from build123d import *

# Parameters (mm, degrees)
BOSS_EXTRUDE1_DEPTH = 4.8
SKETCH2_R           = 8.5
BOSS_EXTRUDE2_DEPTH = 8.5
CUT_EXTRUDE1_DEPTH  = 18.927353402


with BuildPart() as part:
    # Sketch1 → Boss-Extrude1 (new body)
    with BuildSketch(Plane(origin=(0, 0, 0), x_dir=(1, 0, 0), z_dir=(0, 1, 0))):
        Polygon((-6, 3.464101615), (0, 6.92820323), (6, 3.464101615), (6, -3.464101615), (0, -6.92820323), (-6, -3.464101615), align=None)
    extrude(amount=BOSS_EXTRUDE1_DEPTH)

    # Sketch2 → Boss-Extrude2 (add)
    with BuildSketch(Plane(origin=(0, 4.8, 0), x_dir=(1, 0, 0), z_dir=(0, 1, 0))):
        with Locations(Location((0, 0, 0), (0, 0, 270))):
            Circle(SKETCH2_R)
    extrude(amount=BOSS_EXTRUDE2_DEPTH)

    # Sketch3 → Cut-Extrude1 (cut, through all)
    with BuildSketch(Plane(origin=(0, 13.3, 0), x_dir=(1, 0, 0), z_dir=(0, 1, 0))):
        with BuildLine():
            Line((-1.802775638, 3), (1.802775638, 3))
            ThreePointArc((1.802775638, 3), (0, -3.5), (-1.802775638, 3))
        make_face()
    extrude(amount=-CUT_EXTRUDE1_DEPTH, mode=Mode.SUBTRACT)


solid = part.part
Verification items for the finished model (mm, model axes). A direction names the side the tool comes from. Round coordinates to 2 decimals unless told otherwise and drop trailing zeros. Order: outer loops, then holes, each group sorted by start corner. A loop starts at its lowest first (then second) coordinate and runs counter-clockwise, first axis right, second up.
1. Section check B-B on y = 4.5. Record the cut outline in (x, z), then the cut area to 3 significant figures.
Final values:
outline: (-6, -3.46) - (0, -6.93) - (6, -3.46) - (6, 3.46) - (0, 6.93) - (-6, 3.46) - close; hole (-1.8, -3) - (1.8, -3) arc R3.5 ccw (long way) to start
area: 87.4 mm2
2. Thickness scan on L1, parallel to X at y = 8.25, z = 0; L2, parallel to Y at x = 0.25, z = 7; L3, parallel to Z at x = 0.75, y = 12.5. Record the ranges inside material, lowest first.
Final values:
L1: x = -8.5 to -3.5, 3.5 to 8.5
L2: y = 4.8 to 13.3
L3: z = -8.47 to -3, 3.42 to 8.47
3. Section check C-C on x = 2.25. Record the cut outline in (y, z).
Final values:
outline: (0, -5.63) - (4.8, -5.63) - (4.8, -8.2) - (13.3, -8.2) - (13.3, -2.68) - (0, -2.68) - close; (0, 2.68) - (13.3, 2.68) - (13.3, 8.2) - (4.8, 8.2) - (4.8, 5.63) - (0, 5.63) - close
4. Section check A-A on z = 0. Record the cut outline in (x, y), then the cut area to 3 significant figures.
Final values:
outline: (-8.5, 4.8) - (-6, 4.8) - (-6, 0) - (-3.5, 0) - (-3.5, 13.3) - (-8.5, 13.3) - close; (3.5, 0) - (6, 0) - (6, 4.8) - (8.5, 4.8) - (8.5, 13.3) - (3.5, 13.3) - close
area: 109 mm2
5. Access from +Z, -Z, +X, -X, +Y, -Y to the whole of each face (thin tool, end or side, straight path). Record for faces 1 (the flat face through (3.042, 2.366, 5.172)), 2 (the flat face through (-2.96, 2.37, 5.22)), 3 (the flat face through (2.96, 2.37, -5.22)), 4 (the flat face through (-3.042, 2.366, -5.172)).
Final values:
face 1: +Z, +X, -Y
face 2: +Z, -X, -Y
face 3: -Z, +X, -Y
face 4: -Z, -X, -Y
6. Release check for a two-part mould opening along X. For faces 5 (the flat face through (0, 7, -3)), 6 (the cylindrical face through (8.428, 8.99, -1.107)), 7 (the flat face through (-6.3, 4.8, 0)) record: +X half, -X half, draft (parallel to the pull), parting line (faces both ways), or undercut.
Final values:
face 5: undercut
face 6: parting line
face 7: draft
7. Go/stop test with flat-tipped pins: P1, Ø4, axis at y = 1.5, z = -1, coming from the -X side; P2, Ø1.5, axis at y = 11, z = -3.5, coming from the +X side; P3, Ø5, axis at y = 10, z = -4, coming from the -X side. Record where each tip stops, or that it passes through.
Final values:
P1: stops at x = -6
P2: stops at x = 8.04
P3: stops at x = -8.37
8. Section check D-D on x = -5.5. Record the cut outline in (y, z), then the cut area to 3 significant figures.
Final values:
outline: (0, -3.75) - (4.8, -3.75) - (4.8, -6.48) - (13.3, -6.48) - (13.3, 6.48) - (4.8, 6.48) - (4.8, 3.75) - (0, 3.75) - close
area: 146 mm2
